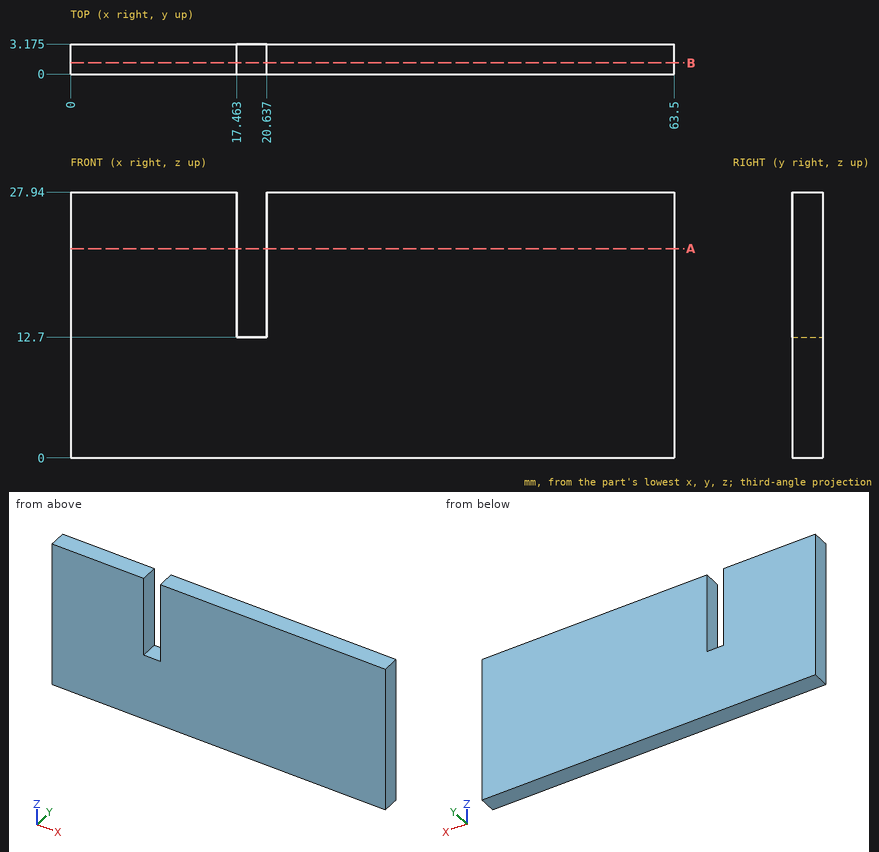
For this review, use the dimensioned drawing (mm, ordinates from the lowest corner) and the shaded views. Coordinates: 2 decimals unless noted, no trailing zeros. Loops run counter-clockwise (first coordinate to the right, second up) from the corner with the lowest first, then second, coordinate; pieces in that order, holes last. Notation, with made-up numbers: (27, 54.5) - (58, 54.5) arc R16 ccw to (58, 61.5) - close; hole circle Ø3 at (-24, 6.5). An arc over 180 degrees is marked (long way). Use one line per item in the form item = value. Start each with the question number.
1) Take a section at B-B (y = 1.2). State the section outline as (x, z) points, plus the area to 3 significant figures.
2) To check wall thickness, follow probe 1 along X at (y, z) = (1, 14.25); probe 2 along Z at (x, y) = (18, 2.65). State the ranges of each line that lie inside material, in increasing order. Write a range as from..to.
3) Take a section at A-A (z = 22). State the section outline as (x, y) points (1 decimal).
4) For pin 1 (1.6 mm diameter, centred on x = 19, y = 1, fed in from +Z), flat-tipped, find the tip position at first contact; note if it passes through.
From the geometry:
q1.outline = (0, 0) - (63.5, 0) - (63.5, 27.94) - (20.64, 27.94) - (20.64, 12.7) - (17.46, 12.7) - (17.46, 27.94) - (0, 27.94) - close
q1.area = 1,730 mm2
q2.probe_1 = 0..17.46, 20.64..63.5
q2.probe_2 = 0..12.7
q3.outline = (0, 0) - (17.5, 0) - (17.5, 3.2) - (0, 3.2) - close; (20.6, 0) - (63.5, 0) - (63.5, 3.2) - (20.6, 3.2) - close
q4.pin_1 = 12.7
